Autodesk Inventor part; units mm, degrees
ref_plane "YZ Plane" through (0, 0, 0) normal (1, 0, 0) x (0, 1, 0)
ref_plane "XZ Plane" through (0, 0, 0) normal (0, 1, 0) x (-1, 0, 0)
ref_plane "XY Plane" through (0, 0, 0) normal (0, 0, 1) x (1, 0, 0)
sketch "Sketch1" plane through (0, 0, 0) normal (0, 0, 1) x (1, 0, 0)
  circle A0 centre (0, 0) radius 7.5
  circle A1 centre (0, 0) radius 1.6
  dimension "d0" = 15
  dimension "d1" = 3.2
extrude "Ydre diameter" add sketch "Sketch1" along normal blind 4.5
sketch "Sketch2" plane through (0, 0, 4.5) normal (0, 0, 1) x (1, 0, 0)
  circle A0 centre (0, 0) radius 5.25
  dimension "d4" = 10.5
extrude "Indre diameter" add sketch "Sketch2" along normal blind 6
fillet "Fillet1" radius 0.5 1 edges at (-5.25, 0, 10.5)
sketch "Sketch3" plane through (0, 0, 4.5) normal (0, 0, -1) x (-1, 0, 0)
  circle A0 centre (0, 0) radius 1.6
extrude "Reducering af indre hul" add sketch "Sketch3" along normal blind 3.5
properties part number "NØD-knap"
Read the model definition and answer for the solid it produces. Units are mm, in the model's axes. A direction names the side the tool comes from. Round coordinates to 2 decimals unless told otherwise and drop trailing zeros. Write each loop counter-clockwise with the first axis right and the second up, starting at its lowest first coordinate (ties: lowest second). Pieces come first, ordered by that corner, then holes.
1. Straight lines are drawn through the part: L1, parallel to Y at x = 0, z = 0.2; L2, parallel to Z at x = -4.5, y = 5.5; L3, parallel to Z at x = -2.5, y = -4.5. For each, find the intervals that lie inside material, in ascending order.
2. The part is cut by section A-A, the plane y = 0. Determine the outline of the cut face in (x, z), then the cut area to 3 significant figures.
3. Determine the mould class of faces 4 (the face through (-1.8, 5.1, 4.5)), 5 (the face through (0, 0, 1)), 6 (the face through (-7.493, -0.33, 2.218)) for opening direction Y: pulls with the +Y half, pulls with the -Y half, needs draft (parallel to the pull), parting line crosses it, or undercut.
4. The part is cut by section C-C, the plane z = 3.75. Determine the outline of the cut face in (x, y).
5. Given pin 1 Ø1.5 at (x, z) = (1.5, 6.5) entering from -Y; pin 2 Ø2.5 at (x, y) = (-0.5, -0.5) entering from -Z; pin 3 Ø1 at (y, z) = (3, 1.5) entering from -X; pin 4 Ø6 at (x, z) = (-6, 3) entering from +Y, each flat-ended and moving along its own axis, determine where each tip first touches the part or whether it passes through.
6. Which of the six approach directions +Z, -Z, +X, -X, +Y, -Y give full straight-line access (tool end or side, diameter ignored) to faces 1 (the face through (-1.27, 0.97, 0.49)), 2 (the face through (5, -1.6, 7.2)), 3 (the face through (0, 2, 0))?
Values:
1. L1: y = -7.5 to -1.6, 1.6 to 7.5
1. L2: z = 0 to 4.5
1. L3: z = 0 to 10.3
2. outline: (-7.5, 0) - (-1.6, 0) - (-1.6, 1) - (1.6, 1) - (1.6, 0) - (7.5, 0) - (7.5, 4.5) - (5.25, 4.5) - (5.25, 10) arc R0.5 ccw to (4.75, 10.5) - (-4.75, 10.5) arc R0.5 ccw to (-5.25, 10) - (-5.25, 4.5) - (-7.5, 4.5) - close
2. area: 127 mm2
3. face 4: needs draft
3. face 5: undercut
3. face 6: parting line crosses it
4. outline: circle Ø15 at (0, 0)
5. pin 1: stops at y = -5.2
5. pin 2: stops at z = 0
5. pin 3: stops at x = -7.07
5. pin 4: stops at y = 6.87
6. face 1: -Z
6. face 2: +Z
6. face 3: -Z, +X, -X, +Y, -Y
